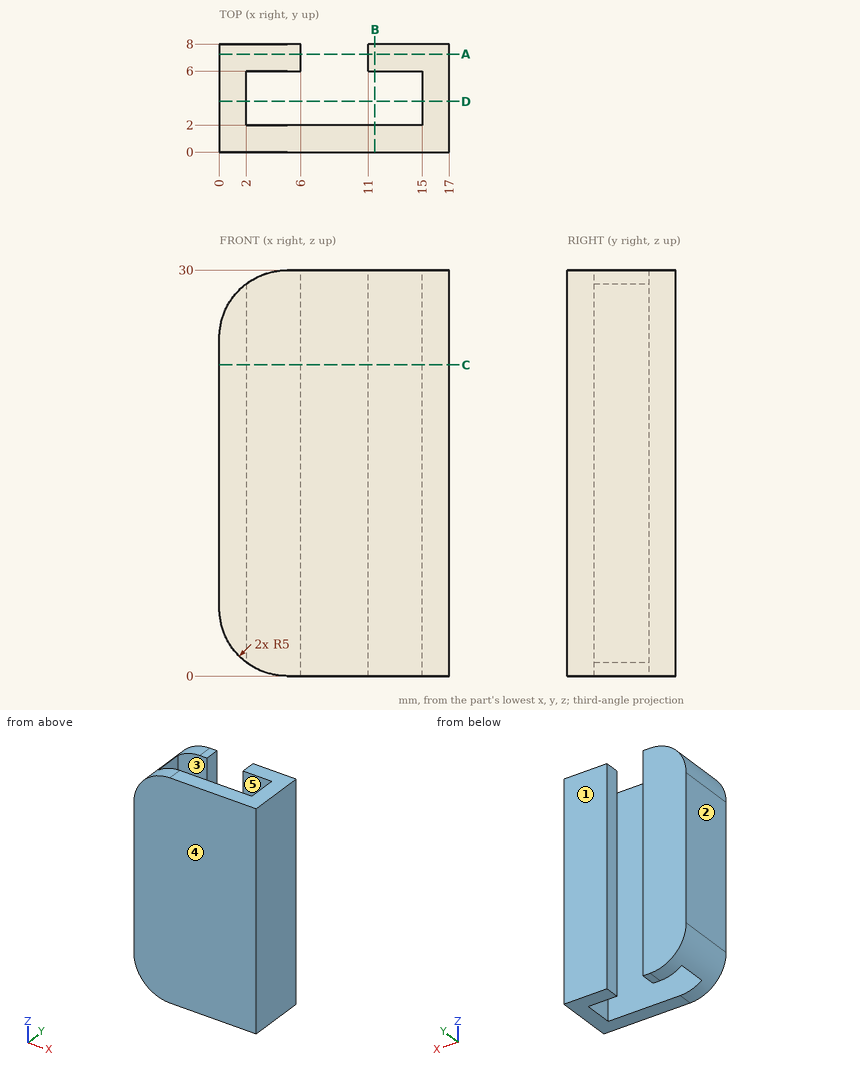
The figure shows three views and two pictorial views of one solid part (mm, origin at its lowest corner). Answer the questions. A direction names the side the tool comes from. Coordinates: 2 decimals unless noted, no trailing zeros. Loops run counter-clockwise (first coordinate to the right, second up) from the corner with the lowest first, then second, coordinate; pieces in that order, holes last. Notation, with made-up numbers: (25, 0.25) -> (48, 0.25) arc R12 cw to (48, 14.25) -> close; hole circle Ø7 at (-35.5, 72.5). An arc over 180 degrees is marked (long way). Return JSON: item names as keys, results as strings. Group by question number.
(1) Which of the six approach directions +Z, -Z, +X, -X, +Y, -Y give full straight-line access (tool end or side, diameter ignored) to the marked faces 4 and 5?
(2) Given pin 1 Ø6 at (x, z) = (8, 23) entering from +Y; pin 2 Ø1.5 at (x, y) = (7, 6.5) entering from -Z; pin 3 Ø1.5 at (x, y) = (3.5, 1) entering from +Z, each flat-ended and moving along its own axis, determine where each tip first touches the part or whether it passes through.
(3) A cutting plane is placed at A-A on y = 7.25. Write down the section's boundary in (x, z).
(4) A cutting plane is placed at C-C on z = 23. Write down the section's boundary in (x, y), and give its area (3 significant figures).
(5) A cutting plane is placed at D-D on y = 3.75. Write down the section's boundary in (x, z), and give its area (3 significant figures).
(6) Find the intervals of material crossed by probe 1 along X at (y, z) = (6.75, 12); probe 2 along X at (y, z) = (5, 21); probe 3 along Y at (x, z) = (12, 17.5), in increasing order. Write a range as from..to.
(7) Determine the mould class of the marked faces 1, 2 and 3 for opening direction X: released by +X, released by -X, zero draft, split by the parting line, or undercut.
(8) A cutting plane is placed at B-B on x = 11.5. Write down the section's boundary in (y, z), and give its area (3 significant figures).
The answers:
{
 "1": {"face 4": "+Z, -Z, +X, -X, -Y", "face 5": "+Z, -Z"},
 "2": {"pin 1": "stops at y = 8", "pin 2": "passes through", "pin 3": "stops at z = 29.94"},
 "3": {"outline": "(0, 5) arc R5 ccw to (5, 0) -> (6, 0) -> (6, 30) -> (5, 30) arc R5 ccw to (0, 25) -> close; (11, 0) -> (17, 0) -> (17, 30) -> (11, 30) -> close"},
 "4": {"outline": "(0, 0) -> (17, 0) -> (17, 8) -> (11, 8) -> (11, 6) -> (15, 6) -> (15, 2) -> (2, 2) -> (2, 6) -> (6, 6) -> (6, 8) -> (0, 8) -> close", "area": "74.0 mm^2"},
 "5": {"outline": "(0, 5) arc R5 ccw to (2, 1) -> (2, 29) arc R5 ccw to (0, 25) -> close; (15, 0) -> (17, 0) -> (17, 30) -> (15, 30) -> close", "area": "111 mm^2"},
 "6": {"probe 1": "x = 0..6, 11..17", "probe 2": "x = 0..2, 15..17", "probe 3": "y = 0..2, 6..8"},
 "7": {"face 1": "zero draft", "face 2": "released by -X", "face 3": "undercut"},
 "8": {"outline": "(0, 0) -> (2, 0) -> (2, 30) -> (0, 30) -> close; (6, 0) -> (8, 0) -> (8, 30) -> (6, 30) -> close", "area": "120 mm^2"}
}
